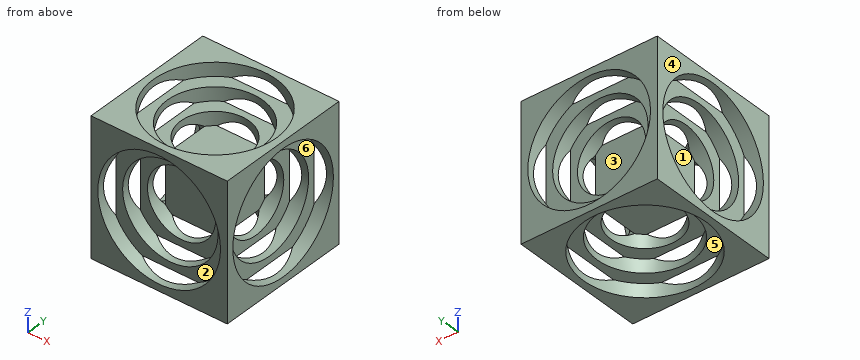
from build123d import *

# Parameters (mm, degrees)
F2_W          = 100
F2_H          = 100
F3_DEPTH      = 50
F3_DEPTH_BACK = 50
F5_R          = 45
F6_DEPTH      = 10
F8_R          = 45
F9_DEPTH      = 10
F11_R         = 45
F12_DEPTH     = 10
F14_R         = 45
F15_DEPTH     = 10
F17_R         = 45
F18_DEPTH     = 10
F20_R         = 45
F21_DEPTH     = 10
F22_R         = 35
F23_DEPTH     = 10
F24_R         = 35
F25_DEPTH     = 10
F26_R         = 35
F27_DEPTH     = 10
F28_R         = 35
F29_DEPTH     = 10
F30_R         = 35
F31_DEPTH     = 10
F32_R         = 35
F33_DEPTH     = 10
F34_R         = 25
F35_DEPTH     = 10
F36_R         = 25
F37_DEPTH     = 10
F38_R         = 25
F39_DEPTH     = 10
F40_R         = 25
F41_DEPTH     = 10
F42_R         = 25
F43_DEPTH     = 10
F44_R         = 25
F45_DEPTH     = 10


with BuildPart() as f3:
    # F2 (on Top) → F3 (new body, two sides)
    with BuildSketch(Plane.XY) as f3_sk:
        Rectangle(F2_W, F2_H)
    extrude(amount=F3_DEPTH)
    extrude(f3_sk.sketch, amount=-F3_DEPTH_BACK)

    # F5 (on offset) → F6 (cut)
    with BuildSketch(Plane.XZ.offset(50)):
        Circle(F5_R)
    extrude(amount=-F6_DEPTH, mode=Mode.SUBTRACT)

    # F8 (on offset) → F9 (cut)
    with BuildSketch(Plane.YZ.offset(50)):
        Circle(F8_R)
    extrude(amount=-F9_DEPTH, mode=Mode.SUBTRACT)

    # F11 (on offset) → F12 (cut)
    with BuildSketch(Plane.XY.offset(50)):
        Circle(F11_R)
    extrude(amount=-F12_DEPTH, mode=Mode.SUBTRACT)

    # F14 (on offset) → F15 (cut)
    with BuildSketch(Plane.XY.offset(-50)):
        Circle(F14_R)
    extrude(amount=F15_DEPTH, mode=Mode.SUBTRACT)

    # F17 (on offset) → F18 (cut)
    with BuildSketch(Plane.XZ.offset(-50)):
        Circle(F17_R)
    extrude(amount=F18_DEPTH, mode=Mode.SUBTRACT)

    # F20 (on offset) → F21 (cut)
    with BuildSketch(Plane.YZ.offset(-50)):
        Circle(F20_R)
    extrude(amount=F21_DEPTH, mode=Mode.SUBTRACT)

    # F22 (on face) → F23 (cut)
    with BuildSketch(Plane(origin=(-40, 0, 0), x_dir=(0, -1, 0), z_dir=(-1, 0, 0))):
        Circle(F22_R)
    extrude(amount=-F23_DEPTH, mode=Mode.SUBTRACT)

    # F24 (on face) → F25 (cut)
    with BuildSketch(Plane.XZ.offset(40)):
        Circle(F24_R)
    extrude(amount=-F25_DEPTH, mode=Mode.SUBTRACT)

    # F26 (on face) → F27 (cut)
    with BuildSketch(Plane.XY.offset(40)):
        Circle(F26_R)
    extrude(amount=-F27_DEPTH, mode=Mode.SUBTRACT)

    # F28 (on face) → F29 (cut)
    with BuildSketch(Plane(origin=(0, 40, 0), x_dir=(-1, 0, 0), z_dir=(0, 1, 0))):
        Circle(F28_R)
    extrude(amount=-F29_DEPTH, mode=Mode.SUBTRACT)

    # F30 (on face) → F31 (cut)
    with BuildSketch(Plane(origin=(0, 0, -40), x_dir=(1, 0, 0), z_dir=(0, 0, -1))):
        Circle(F30_R)
    extrude(amount=-F31_DEPTH, mode=Mode.SUBTRACT)

    # F32 (on face) → F33 (cut)
    with BuildSketch(Plane.YZ.offset(40)):
        Circle(F32_R)
    extrude(amount=-F33_DEPTH, mode=Mode.SUBTRACT)

    # F34 (on face) → F35 (cut)
    with BuildSketch(Plane.XZ.offset(30)):
        Circle(F34_R)
    extrude(amount=-F35_DEPTH, mode=Mode.SUBTRACT)

    # F36 (on face) → F37 (cut)
    with BuildSketch(Plane(origin=(0, 0, -30), x_dir=(1, 0, 0), z_dir=(0, 0, -1))):
        Circle(F36_R)
    extrude(amount=-F37_DEPTH, mode=Mode.SUBTRACT)

    # F38 (on face) → F39 (cut)
    with BuildSketch(Plane(origin=(0, 30, 0), x_dir=(-1, 0, 0), z_dir=(0, 1, 0))):
        Circle(F38_R)
    extrude(amount=-F39_DEPTH, mode=Mode.SUBTRACT)

    # F40 (on face) → F41 (cut)
    with BuildSketch(Plane.XY.offset(30)):
        Circle(F40_R)
    extrude(amount=-F41_DEPTH, mode=Mode.SUBTRACT)

    # F42 (on face) → F43 (cut)
    with BuildSketch(Plane.YZ.offset(30)):
        Circle(F42_R)
    extrude(amount=-F43_DEPTH, mode=Mode.SUBTRACT)

    # F44 (on face) → F45 (cut)
    with BuildSketch(Plane(origin=(-30, 0, 0), x_dir=(0, -1, 0), z_dir=(-1, 0, 0))):
        Circle(F44_R)
    extrude(amount=-F45_DEPTH, mode=Mode.SUBTRACT)


solid = f3.part
Input: part model. Units: mm. Frame: model coordinates. Face numbers are marked on the shaded views. A direction names the side the tool comes from. Coordinates: 2 decimals unless noted, no trailing zeros. Loops run counter-clockwise (first coordinate to the right, second up) from the corner with the lowest first, then second, coordinate; pieces in that order, holes last. Notation, with made-up numbers: (-24.75, -20.75) -> (-17.75, -20.75) arc R6 ccw to (-17.75, -15.75) -> close; hole circle Ø11 at (27.25, -1). An arc over 180 degrees is marked (long way). Write each question's results on one line, items separated by ' | '. Start each with the question number.
Q1. Ray query, line 1 (X direction, y = 45.5, z = 0); line 2 (Y direction, x = 0, z = 27). Return the intervals inside material, ascending. Write a range as from..to.
Q2. Reachability of the marked faces 1, 2 and 3 from +Z, -Z, +X, -X, +Y, -Y: full face, straight path, thin tool, end or side. Return the list, or none.
Q3. Pull-direction query (Z, two-part tool) for the marked faces 4, 5 and 6; classes: released by +Z, released by -Z, zero draft, split by the parting line, or undercut.
Q4. Section B-B, the plane y = 0. State how many separate pieces and enclosed holes the cut face has, plus the area to 3 significant figures.
Q5. Section A-A, the plane y = -42.5. Return the cut outline in (x, z).
Q6. Pin query (flat end, axial travel): pin 1 (8 mm diameter, centred on y = -12.5, z = 5.5, fed in from +X); pin 2 (2 mm diameter, centred on x = 15.5, z = 37, fed in from +Y); pin 3 (8 mm diameter, centred on x = -3.5, y = -11.5, fed in from +Z). Return the tip coordinate at first contact, or that it passes through.
Found:
1) line 1: -50..-45, 45..50 | line 2: -30..-25, 25..30
2) face 1: -X | face 2: -Y | face 3: +Y
3) face 4: zero draft | face 5: released by -Z | face 6: undercut
4) separate pieces: 13 | enclosed holes: 0 | area: 1,900 mm2
5) outline: (-50, -50) -> (-14.79, -50) -> (-14.79, -42.5) arc R45 cw to (-42.5, -14.79) -> (-50, -14.79) -> close; (-50, 14.79) -> (-42.5, 14.79) arc R45 cw to (-14.79, 42.5) -> (-14.79, 50) -> (-50, 50) -> close; (14.79, -50) -> (50, -50) -> (50, -14.79) -> (42.5, -14.79) arc R45 cw to (14.79, -42.5) -> close; (14.79, 42.5) arc R45 cw to (42.5, 14.79) -> (50, 14.79) -> (50, 50) -> (14.79, 50) -> close
6) pin 1: x = 20 | pin 2: y = 40 | pin 3: z = 20
